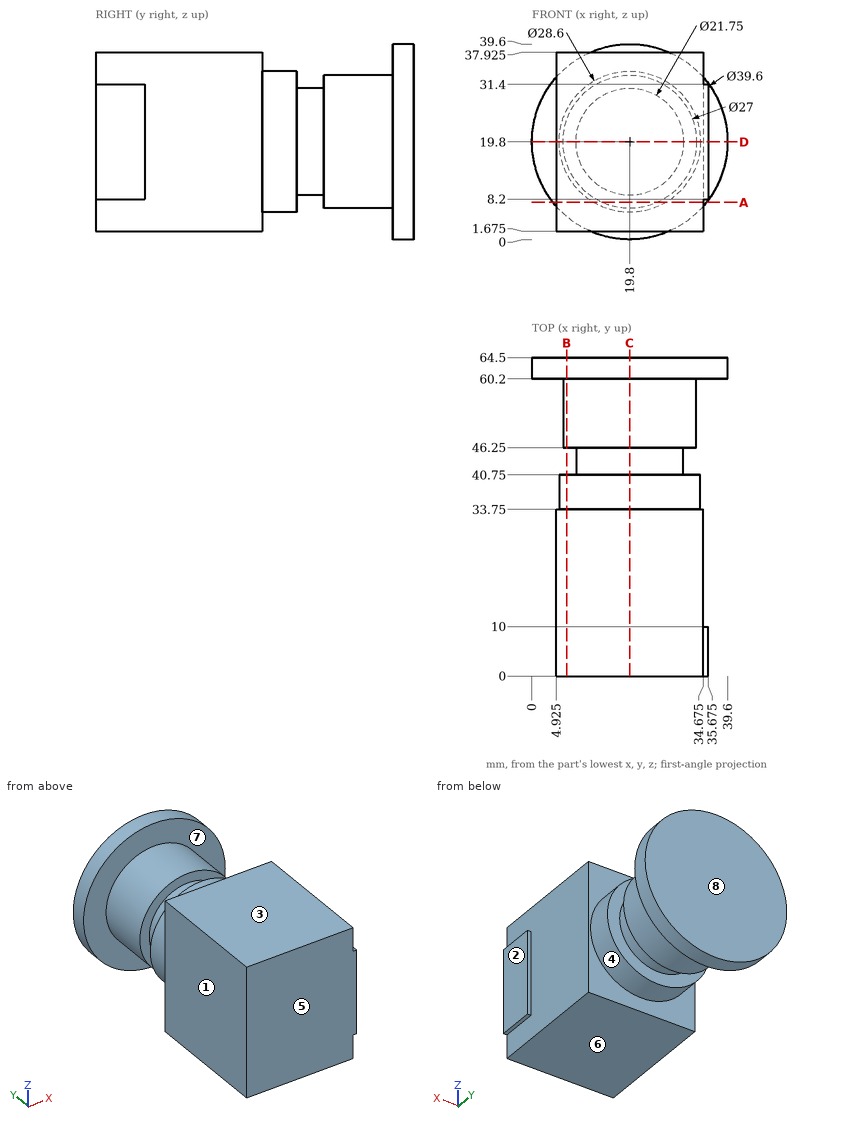
Design review of the part shown in the three views and the two pictorial views. Dimensions are in mm from the part's minimum x, y and z. A direction names the side the tool comes from. Give positions to 0.01 mm unless a question says otherwise; leave off trailing zeros. Loops run counter-clockwise (first coordinate to the right, second up) from the corner with the lowest first, then second, coordinate; pieces in that order, holes last. Notation, with made-up numbers: (-15.75, -7) -> (6.25, -7) arc R24 ccw to (6.25, 28) -> close; hole circle Ø1 at (-11.75, -7.5). An arc over 180 degrees is marked (long way). Put each result on its own line as item: value. Start each with the question number.
1. We need section B-B on x = 7. State the section outline as (y, z) points (3 decimals), then the cut area to 3 significant figures.
2. We need section C-C on x = 19.8. State the section outline as (y, z) points (3 decimals), then the cut area to 3 significant figures.
3. We need section A-A on z = 7.5. State the section outline as (x, y) points (3 decimals).
4. We need section D-D on z = 19.8. State the section outline as (x, y) points (3 decimals), then the cut area to 3 significant figures.
5. For the marked faces 1, 2, 3 and 4, list the 3-axis set-ups (+Z, -Z, +X, -X, +Y, -Y) from which the entire face can be reached by the end or side of a thin tool; tool diameter is ignored.
6. Clearance check with flat-ended pins moving along their axes: P1, Ø5, axis at y = 53.5, z = 25, coming from the -X side; P2, Ø17, axis at y = 19.5, z = 12, coming from the -X side (3 decimals); P3, Ø10, axis at y = 23, z = 23.5, coming from the +X side (3 decimals). State where each tip first meets the part, or that it passes through.
7. Wall thickness on probe 1 along Y at (x, z) = (17.5, 6); probe 2 along Y at (x, z) = (26.5, 32.5); probe 3 along Z at (x, y) = (20, 20.5) (3 decimals): over which ranges is each line inside the solid? List them lowest first.
8. Mouldability with a two-part tool opening along Y and no side actions: class the marked faces 5, 6, 7 and 8 as released by +Y, released by -Y, zero draft, split by the parting line, or undercut.
Determined:
1. outline: (0, 1.675) -> (33.75, 1.675) -> (33.75, 13.424) -> (40.75, 13.424) -> (40.75, 26.176) -> (33.75, 26.176) -> (33.75, 37.925) -> (0, 37.925) -> close; (46.25, 15.509) -> (60.2, 15.509) -> (60.2, 4.694) -> (64.5, 4.694) -> (64.5, 34.906) -> (60.2, 34.906) -> (60.2, 24.091) -> (46.25, 24.091) -> close
1. area: 1,560 mm^2
2. outline: (0, 1.675) -> (33.75, 1.675) -> (33.75, 5.5) -> (40.75, 5.5) -> (40.75, 8.925) -> (46.25, 8.925) -> (46.25, 6.3) -> (60.2, 6.3) -> (60.2, 0) -> (64.5, 0) -> (64.5, 39.6) -> (60.2, 39.6) -> (60.2, 33.3) -> (46.25, 33.3) -> (46.25, 30.675) -> (40.75, 30.675) -> (40.75, 34.1) -> (33.75, 34.1) -> (33.75, 37.925) -> (0, 37.925) -> close
2. area: 2,090 mm^2
3. outline: (4.284, 60.2) -> (14.236, 60.2) -> (14.236, 46.25) -> (25.364, 46.25) -> (25.364, 60.2) -> (35.316, 60.2) -> (35.316, 64.5) -> (4.284, 64.5) -> close; (4.925, 0) -> (34.675, 0) -> (34.675, 33.75) -> (27.094, 33.75) -> (27.094, 40.75) -> (12.506, 40.75) -> (12.506, 33.75) -> (4.925, 33.75) -> close
4. outline: (0, 60.2) -> (6.3, 60.2) -> (6.3, 46.25) -> (8.925, 46.25) -> (8.925, 40.75) -> (5.5, 40.75) -> (5.5, 33.75) -> (4.925, 33.75) -> (4.925, 0) -> (35.675, 0) -> (35.675, 10) -> (34.675, 10) -> (34.675, 33.75) -> (34.1, 33.75) -> (34.1, 40.75) -> (30.675, 40.75) -> (30.675, 46.25) -> (33.3, 46.25) -> (33.3, 60.2) -> (39.6, 60.2) -> (39.6, 64.5) -> (0, 64.5) -> close
4. area: 1,880 mm^2
5. face 1: +Z, -Z, -X, -Y
5. face 2: +Z, -Z, +X, -Y
5. face 3: +Z, +X, -X, -Y
5. face 4: none
6. P1: x = 6.57
6. P2: x = 4.925
6. P3: x = 34.675
7. probe 1: 0 to 40.75, 60.2 to 64.5
7. probe 2: 0 to 33.75, 60.2 to 64.5
7. probe 3: 1.675 to 37.925
8. face 5: released by -Y
8. face 6: zero draft
8. face 7: undercut
8. face 8: released by +Y
